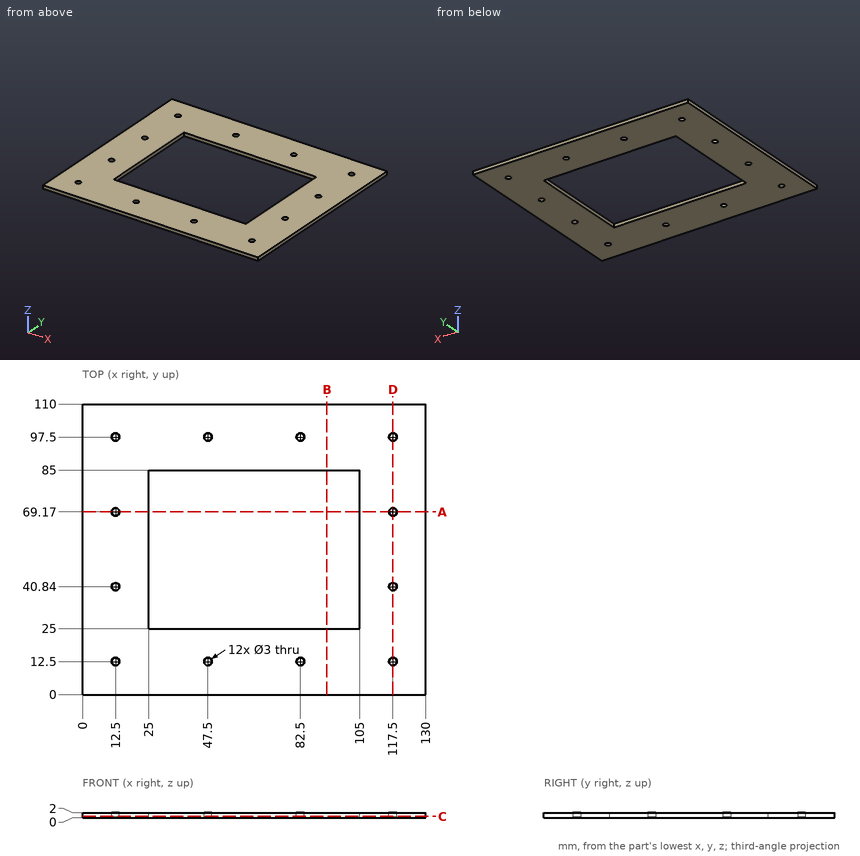
Answer from the drawing. Dimensions are ordinates in mm from the lowest x, y and z of the part. Coordinates: 2 decimals unless noted, no trailing zeros. Write each loop counter-clockwise with the first axis right and the second up, starting at its lowest first coordinate (ties: lowest second). Pieces come first, ordered by that corner, then holes. Notation, with made-up numbers: (-8, 1) - (6, 1) arc R19 ccw to (6, 15) - close; hole circle Ø8 at (77, 19.5). An arc over 180 degrees is marked (long way). Return JSON: item names as keys, results as strings. Group by question number.
Q1. Find the intervals of material crossed by line 1 along Y through (x, z) = (12.5, 0.7); line 2 along Y through (x, z) = (47.5, 0.9); line 3 along X through (y, z) = (40.84, 1.5), in increasing order. Write a range as [from, to].
Q2. The part is cut by section C-C on z = 0.6. State how many separate pieces and enclosed holes the cut face has, and give its area (3 significant figures).
Q3. The part is cut by section B-B on x = 92.5. Write down the section's boundary in (y, z).
Q4. The part is cut by section A-A on y = 69.17. Write down the section's boundary in (x, z), and give its area (3 significant figures).
Q5. The part is cut by section D-D on x = 117.5. Write down the section's boundary in (y, z), and give its area (3 significant figures).
Evaluation:
{
 "1": {"line 1": "y = [0, 11], [14, 39.34], [42.34, 67.67], [70.67, 96], [99, 110]", "line 2": "y = [0, 11], [14, 25], [85, 96], [99, 110]", "line 3": "x = [0, 11], [14, 25], [105, 116], [119, 130]"},
 "2": {"separate pieces": "1", "enclosed holes": "13", "area": "9,420 mm2"},
 "3": {"outline": "(0, 0) - (25, 0) - (25, 2) - (0, 2) - close; (85, 0) - (110, 0) - (110, 2) - (85, 2) - close"},
 "4": {"outline": "(0, 0) - (11, 0) - (11, 2) - (0, 2) - close; (14, 0) - (25, 0) - (25, 2) - (14, 2) - close; (105, 0) - (116, 0) - (116, 2) - (105, 2) - close; (119, 0) - (130, 0) - (130, 2) - (119, 2) - close", "area": "88.0 mm2"},
 "5": {"outline": "(0, 0) - (11, 0) - (11, 2) - (0, 2) - close; (14, 0) - (39.34, 0) - (39.34, 2) - (14, 2) - close; (42.34, 0) - (67.67, 0) - (67.67, 2) - (42.34, 2) - close; (70.67, 0) - (96, 0) - (96, 2) - (70.67, 2) - close; (99, 0) - (110, 0) - (110, 2) - (99, 2) - close", "area": "196 mm2"}
}
